Input: part model. Units: mm. Frame: model coordinates. Face numbers are marked on the shaded views. A direction names the side the tool comes from. Coordinates: 2 decimals unless noted, no trailing zeros. Order: outer loops, then holes, each group sorted by start corner. A loop starts at its lowest first (then second) coordinate and runs counter-clockwise, first axis right, second up. Notation, with made-up numbers: (-22.75, 79) -> (-10.75, 79) arc R28 cw to (-10.75, 102) -> close; hole circle Ø6 at (63, 39). An arc over 180 degrees is marked (long way). Answer as CSV lines item,"result".
from build123d import *


with BuildPart() as part:
    # Esquisse1 → Révolution1 (revolve)
    with BuildSketch(Plane(origin=(0, 0, 0), x_dir=(1, 0, 0), z_dir=(0, 1, 0))):
        Polygon((3, 2), (3, -3), (3.5, -3.5), (4, -3.5), (4.5, -3), (4.5, -2.5), (6, -2.5), (6.5, -2), (6.5, 2), (6, 2.5), (3.5, 2.5), align=None)
    revolve(axis=Axis((0, 0, 3.5), (0, 0, -1)))

    # Esquisse2 → Enlèvement de matière-Révolution1 (revolve, cut)
    with BuildSketch(Plane.XY, mode=Mode.PRIVATE) as enl_vement_de_mati_re_r_volution1_sk:
        Polygon((2, 0), (2, 1.2295), (6.2295, 1.2295), (6.5, 1.5), (6.5, 0), align=None)
    revolve(enl_vement_de_mati_re_r_volution1_sk.sketch.rotate(Axis((6.5, 0, 0), (-1, 0, 0)), 90), axis=Axis((6.5, 0, 0), (-1, 0, 0)), mode=Mode.SUBTRACT)

    # Esquisse3 → Enlèvement de matière-Révolution2 (revolve, cut)
    with BuildSketch(Plane.XY):
        Polygon((0, 2), (-1.2295, 2), (-1.2295, 6.2295), (-1.5, 6.5), (0, 6.5), align=None)
    revolve(axis=Axis((0, 6.5, 0), (0, -1, 0)), mode=Mode.SUBTRACT)


solid = part.part
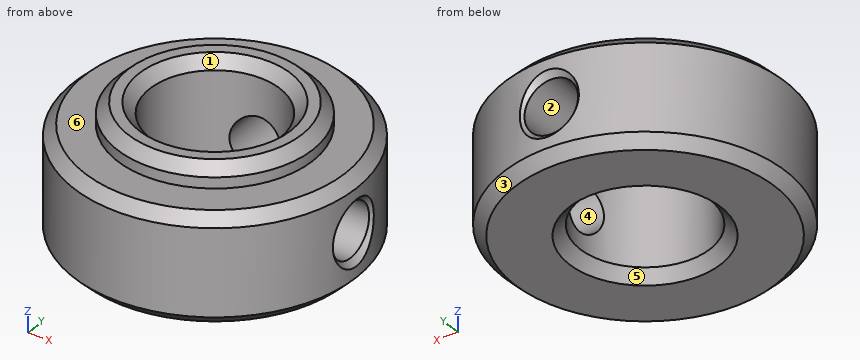
1. Mould query, pull axis Z, two halves, no side actions, for the marked faces 1, 2 and 3. Classes: released by +Z, released by -Z, zero draft, split by the parting line, or undercut.
Findings:
face 1,"released by +Z"
face 2,"undercut"
face 3,"released by -Z"
2. Reachability of the marked faces 4, 5 and 6 from +Z, -Z, +X, -X, +Y, -Y: full face, straight path, thin tool, end or side. Return the list, or none.
Findings:
face 4,"+X"
face 5,"-Z"
face 6,"+Z"
3. Cut plane A-A (y = 0). Return the cut outline in (x, z), plus the area to 3 significant figures.
Findings:
outline,"(-6.5, -2) -> (-6, -2.5) -> (-3.5, -2.5) -> (-3, -2) -> (-3, 3) -> (-3.5, 3.5) -> (-4, 3.5) -> (-4.5, 3) -> (-4.5, 2.5) -> (-6, 2.5) -> (-6.5, 2) -> close; (3, -2) -> (3.5, -2.5) -> (6, -2.5) -> (6.5, -2) -> (6.5, -1.5) -> (6.23, -1.23) -> (3, -1.23) -> close; (3, 1.23) -> (6.23, 1.23) -> (6.5, 1.5) -> (6.5, 2) -> (6, 2.5) -> (4.5, 2.5) -> (4.5, 3) -> (4, 3.5) -> (3.5, 3.5) -> (3, 3) -> close"
area,"28.1 mm2"
4. Cut plane C-C (z = 0). Return the cut outline in (x, y).
Findings:
outline,"(-1.36, 6.36) arc R6.5 ccw (long way) to (6.36, -1.36) -> (6.23, -1.23) -> (2.74, -1.23) arc R3 cw (long way) to (-1.23, 2.74) -> (-1.23, 6.23) -> close; (1.23, 2.74) arc R3 cw to (2.74, 1.23) -> (6.23, 1.23) -> (6.36, 1.36) arc R6.5 ccw to (1.36, 6.36) -> (1.23, 6.23) -> close"
5. Ray query, line 1 along X through (y, z) = (0, 1.6); line 2 along Z through (x, y) = (0, 5.3); line 3 along Z through (x, y) = (0, 3.75). Return the intervals inside material, ascending.
Findings:
line 1,"x = -6.5 to -3, 3 to 6.5"
line 2,"z = -2.5 to -1.23, 1.23 to 2.5"
line 3,"z = -2.5 to -1.23, 1.23 to 3.5"
6. Contact query for flat-ended pins moving along their axis: pin 1 (2 mm diameter, centred on x = 1, z = 0, fed in from +Y); pin 2 (1.5 mm diameter, centred on x = -2.5, z = 0.5, fed in from +Y); pin 3 (1.5 mm diameter, centred on x = -4, z = 0.5, fed in from -Y). Output: stop coordinate, or through.
Findings:
pin 1,"stops at y = 6.42"
pin 2,"stops at y = 6.26"
pin 3,"stops at y = -5.63"
